Source: CAD feature listing. Evaluate the final solid. Frame: model axes, mm. A direction names the side the tool comes from. Round coordinates to 2 decimals unless told otherwise and drop trailing zeros. Loops run counter-clockwise (first coordinate to the right, second up) from the corner with the lowest first, then second, coordinate; pieces in that order, holes last. Notation, with made-up numbers: M -19,75 L -12,75 A9 cw -12,85 Z; hole C 17.5,23 d8. An arc over 180 degrees is marked long. One line per item, written item: value.
from build123d import *

# Parameters (mm, degrees)
SKIZZE2_R         = 43.75
ZAHNFL_CHE_DEPTH  = 6
SKIZZE4_R         = 45.25
SEITENTEIL1_DEPTH = 2
SEITENTEIL2_START = 2
SKIZZE5_R         = 45.25
SEITENTEIL2_DEPTH = 2
AUSSPARUNG_DEPTH  = 65.769784622


with BuildPart() as part:
    # Skizze2 → Zahnfläche (new body)
    with BuildSketch(Plane.XY):
        Circle(SKIZZE2_R)
    extrude(amount=ZAHNFL_CHE_DEPTH)

    # Skizze4 → Seitenteil1 (add)
    with BuildSketch(Plane(origin=(0, 0, 0), x_dir=(-1, 0, 0), z_dir=(0, 0, -1))):
        Circle(SKIZZE4_R)
    extrude(amount=SEITENTEIL1_DEPTH)

    # Skizze5 → Seitenteil2 (add)
    with BuildSketch(Plane.XY.offset(6).offset(SEITENTEIL2_START)):
        with Locations(Location((0, 0, 0), (0, 0, 180))):
            Circle(SKIZZE5_R)
    extrude(amount=-SEITENTEIL2_DEPTH)

    # Skizze6 → Aussparung (cut, through all)
    with BuildSketch(Plane.XY.offset(8)):
        with BuildLine():
            Line((-1.089724736, 2.25), (1.089724736, 2.25))
            ThreePointArc((1.089724736, 2.25), (0, -2.5), (-1.089724736, 2.25))
        make_face()
    extrude(amount=-AUSSPARUNG_DEPTH, mode=Mode.SUBTRACT)


solid = part.part
1. Section query D-D (x = -24.5). Return the cut outline in (y, z), and give its area (3 significant figures).
Report:
outline: M -38.04,-2 L 38.04,-2 L 38.04,0 L 36.25,0 L 36.25,6 L 38.04,6 L 38.04,8 L -38.04,8 L -38.04,6 L -36.25,6 L -36.25,0 L -38.04,0 Z
area: 739 mm2
2. Reachability of faces 4 (the face through (0, 2.25, 3)), 5 (the face through (-32.246, 29.568, 2.958)), 6 (the face through (1, 9, 8)) from +Z, -Z, +X, -X, +Y, -Y: full face, straight path, thin tool, end or side. Return the list, or none.
Report:
face 4: +Z, -Z
face 5: none
face 6: +Z, +X, -X, +Y, -Y
3. Pull-direction query (X, two-part tool) for faces 1 (the face through (0.1, -2.5, 3.1)), 2 (the face through (24, -37, 6)), 3 (the face through (-43.16, 13.59, -0.99)); classes: released by +X, released by -X, zero draft, split by the parting line, or undercut.
Report:
face 1: undercut
face 2: zero draft
face 3: split by the parting line
4. Ray query, line 1 (Y direction, x = 0, z = 3); line 2 (Z direction, x = 40.5, y = -17.5); line 3 (X direction, y = -30, z = 7). Return the intervals inside material, ascending. Write a range as [from, to].
Report:
line 1: y = [-43.75, -2.5], [2.25, 43.75]
line 2: z = [-2, 0], [6, 8]
line 3: x = [-33.88, 33.88]
5. Section query B-B (x = 0). Return the cut outline in (y, z), and give its area (4 significant figures).
Report:
outline: M -45.25,-2 L -2.5,-2 L -2.5,8 L -45.25,8 L -45.25,6 L -43.75,6 L -43.75,0 L -45.25,0 Z; M 2.25,-2 L 45.25,-2 L 45.25,0 L 43.75,0 L 43.75,6 L 45.25,6 L 45.25,8 L 2.25,8 Z
area: 839.5 mm2
6. Section query C-C (z = 3.25). Return the cut outline in (x, y).
Report:
outline: C 0,0 d87.5; hole M -1.09,2.25 A2.5 ccw long 1.09,2.25 Z
7. Section query A-A (y = 0). Return the cut outline in (x, z), and give its area (3 significant figures).
Report:
outline: M -45.25,-2 L -2.5,-2 L -2.5,8 L -45.25,8 L -45.25,6 L -43.75,6 L -43.75,0 L -45.25,0 Z; M 2.5,-2 L 45.25,-2 L 45.25,0 L 43.75,0 L 43.75,6 L 45.25,6 L 45.25,8 L 2.5,8 Z
area: 837 mm2
8. Pin query (flat end, axial travel): pin 1 (4 mm diameter, centred on x = -31.5, z = 2.5, fed in from -Y); pin 2 (6 mm diameter, centred on x = 8.5, z = 6.5, fed in from +Y); pin 3 (3 mm diameter, centred on x = -12.5, z = 6, fed in from -Y). Return the tip coordinate at first contact, or that it passes through.
Report:
pin 1: stops at y = -32.31
pin 2: stops at y = 44.91
pin 3: stops at y = -43.89
